Source: CAD feature listing. Evaluate the final solid. Frame: model axes, mm. Face numbers are marked on the shaded views. A direction names the side the tool comes from. Coordinates: 2 decimals unless noted, no trailing zeros. Order: outer loops, then holes, each group sorted by start corner. A loop starts at its lowest first (then second) coordinate and runs counter-clockwise, first axis right, second up. Notation, with made-up numbers: (14, -23.75) -> (31, -23.75) arc R17 cw to (31, 1.25) -> close; hole circle Ø3 at (37.25, -10.5). An arc over 180 degrees is marked (long way). Write item = value, one per line. Start each with the question number.
Item 1: Section query A-A (y = 8). Output: boundary loops of the cut face in (x, z).
Item 2: Contact query for flat-ended pins moving along their axis: pin 1 (6.5 mm diameter, centred on y = 6, z = 3, fed in from +X); pin 2 (2.5 mm diameter, centred on x = 12.5, z = 5.5, fed in from +Y); pin 3 (3.5 mm diameter, centred on x = 11, z = 6.5, fed in from +Y); pin 4 (2.5 mm diameter, centred on y = 7, z = 7, fed in from -X). Output: stop coordinate, or through.
Item 3: Mould query, pull axis X, two halves, no side actions, for the marked faces 1, 2 and 3. Classes: released by +X, released by -X, zero draft, split by the parting line, or undercut.
Item 4: Section query B-B (z = 5.5). Output: boundary loops of the cut face in (x, y), then the cut area to 3 significant figures.
Item 5: Section query D-D (x = -3.5). Output: boundary loops of the cut face in (y, z), then the cut area to 3 significant figures.
Item 6: Ray query, line 1 along Z through (x, y) = (12.5, 0.6); line 2 along X through (y, z) = (6, 5); line 3 along Y through (x, z) = (11, 10.25). Return the intervals inside material, ascending. Write a range as [from, to].
Item 7: Section query C-C (x = 12.5). Output: boundary loops of the cut face in (y, z), then the cut area to 3 significant figures.
Item 8: Set-up query: the marked faces 4, 5 and 6. Return all of +Z, -Z, +X, -X, +Y, -Y with unobstructed straight access to the full face (end or side cutting, diameter ignored); none if empty.
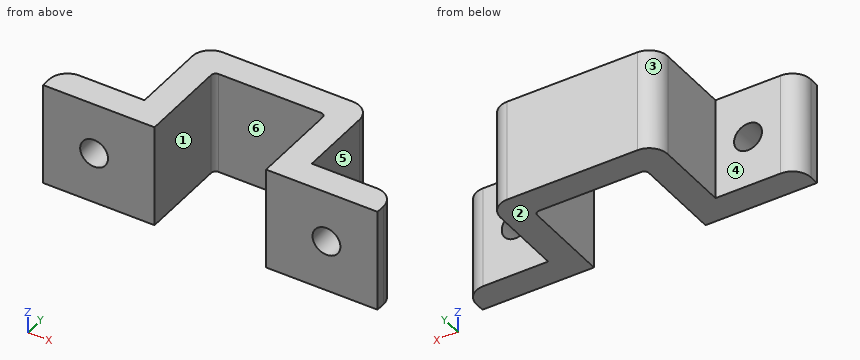
```python
from build123d import *

# Parameters (mm, degrees)
BOSS_EXTRUDE1_DEPTH = 11
FILLET1_R           = 2
FILLET2_R           = 0.5
SKETCH2_R           = 1.5
CUT_EXTRUDE1_DEPTH  = 3


with BuildPart() as part:
    # Sketch1 → Boss-Extrude1 (new body)
    with BuildSketch(Plane.XY):
        Polygon((6, 10), (-6, 10), (-6, 0), (-18, 0), (-18, 3), (-9, 3), (-9, 13), (9, 13), (9, 3), (18, 3), (18, 0), (6, 0), align=None)
    extrude(amount=BOSS_EXTRUDE1_DEPTH)

    # Fillet1
    fillet1_edges = [part.edges().sort_by_distance(p)[0] for p in [
        (-18, 3, 5.5),
        (-9, 13, 5.5),
        (9, 13, 5.5),
        (18, 3, 5.5),
    ]]
    fillet(fillet1_edges, radius=FILLET1_R)

    # Fillet2
    fillet2_edges = [part.edges().sort_by_distance(p)[0] for p in [
        (6, 10, 5.5),
        (-6, 10, 5.5),
    ]]
    fillet(fillet2_edges, radius=FILLET2_R)

    # Sketch2 → Cut-Extrude1 (cut)
    with BuildSketch(Plane(origin=(0, 3, 0), x_dir=(1, 0, 0), z_dir=(0, 1, 0))):
        with Locations(Location((-12.5, -5.5, 0), (0, 0, 270))):
            Circle(SKETCH2_R)
        with Locations(Location((12.5, -5.5, 0), (0, 0, 180))):
            Circle(SKETCH2_R)
    extrude(amount=-CUT_EXTRUDE1_DEPTH, mode=Mode.SUBTRACT)


solid = part.part
```
Computed:
q1.outline = (-9, 0) -> (-6, 0) -> (-6, 11) -> (-9, 11) -> close; (6, 0) -> (9, 0) -> (9, 11) -> (6, 11) -> close
q2.pin_1 = 16.97
q2.pin_2 = through
q2.pin_3 = 3
q2.pin_4 = -9
q3.face_1 = undercut
q3.face_2 = zero draft
q3.face_3 = released by -X
q4.outline = (-18, 0) -> (-14, 0) -> (-14, 3) -> (-16, 3) arc R2 ccw to (-18, 1) -> close; (-11, 0) -> (-6, 0) -> (-6, 9.5) arc R0.5 cw to (-5.5, 10) -> (5.5, 10) arc R0.5 cw to (6, 9.5) -> (6, 0) -> (11, 0) -> (11, 3) -> (9, 3) -> (9, 11) arc R2 ccw to (7, 13) -> (-7, 13) arc R2 ccw to (-9, 11) -> (-9, 3) -> (-11, 3) -> close; (14, 0) -> (18, 0) -> (18, 1) arc R2 ccw to (16, 3) -> (14, 3) -> close
q4.area = 147 mm^2
q5.outline = (10, 0) -> (13, 0) -> (13, 11) -> (10, 11) -> close
q5.area = 33.0 mm^2
q6.line_1 = [0, 4], [7, 11]
q6.line_2 = [-9, -6], [6, 9]
q6.line_3 = [0, 3]
q7.outline = (0, 0) -> (3, 0) -> (3, 4) -> (0, 4) -> close; (0, 7) -> (3, 7) -> (3, 11) -> (0, 11) -> close
q7.area = 24.0 mm^2
q8.face_4 = +Z, -Z, -X, +Y
q8.face_5 = +Z, -Z, +X, +Y
q8.face_6 = +Z, -Z, -Y
